CAD build for the part. Positions are in the model's coordinates, mm. A direction names the side the tool comes from. Give positions to 0.01 mm unless a question says otherwise; leave off trailing zeros. Order: outer loops, then holes, each group sorted by start corner. A loop starts at its lowest first (then second) coordinate and runs counter-clockwise, first axis right, second up.
Item 1: Band-saw the part on C-C on z = -0.5. Give the cut face in (x, y).
Item 2: Band-saw the part on D-D on y = 5. Give the cut face in (x, z).
Item 3: Wall check: L1, parallel to Z at x = -1.5, y = -9.5; L2, parallel to Z at x = 4, y = 0.25; L3, parallel to Y at x = -4, z = -4. Give the ranges that are in metal, low to high.
Item 4: Band-saw the part on A-A on y = 0. Give the cut face in (x, z), plus the area to 3 significant figures.
Item 5: Which spindle directions (+Z, -Z, +X, -X, +Y, -Y) get a long thin tool onto all of the face, cutting with end or side? Do faces 1 (the cylindrical face through (1.764, -3.391, 1.377)), 2 (the flat face through (0, 0, -5.588)). Say none if no direction does.
Item 6: Flat gauge pins, fed straight in: P1, Ø2, axis at x = 6.5, z = 0, coming from the +Y side; P2, Ø3, axis at y = -8, z = -2.5, coming from the -X side; P3, Ø1.5, axis at x = -3, z = -4.5, coming from the +Y side; P4, Ø1, axis at y = -6.5, z = 1.5, coming from the -X side. Where does each tip first touch, or does it go through?
```python
from build123d import *

# Parameters (mm, degrees)
F0_R     = 3.8227
F1_DEPTH = 2.794
F0_R_2   = 6.858
F2_DEPTH = 2.794
F3_R     = 11.3665
F3_R_2   = 6.858
F4_DEPTH = 2.794


with BuildPart() as f1:
    # F0 (on Top) → F1 (new body)
    with BuildSketch(Plane.XY):
        Circle(F0_R)
    extrude(amount=F1_DEPTH)

    # F0 (on Top) → F2 (join)
    with BuildSketch(Plane.XY):
        Circle(F0_R_2)
        Circle(F0_R, mode=Mode.SUBTRACT)
        Circle(F0_R)
    extrude(amount=-F2_DEPTH)

    # F3 (on face) → F4 (join)
    with BuildSketch(Plane(origin=(0, 0, -2.794), x_dir=(1, 0, 0), z_dir=(0, 0, -1))):
        Circle(F3_R)
        Circle(F3_R_2, mode=Mode.SUBTRACT)
        Circle(F3_R_2)
    extrude(amount=F4_DEPTH)


solid = f1.part
```
The answers:
1. outline: circle Ø13.72 at (0, 0)
2. outline: (-10.21, -5.59) - (10.21, -5.59) - (10.21, -2.79) - (4.69, -2.79) - (4.69, 0) - (-4.69, 0) - (-4.69, -2.79) - (-10.21, -2.79) - close
3. L1: z = -5.59 to -2.79
3. L2: z = -5.59 to 0
3. L3: y = -10.64 to 10.64
4. outline: (-11.37, -5.59) - (11.37, -5.59) - (11.37, -2.79) - (6.86, -2.79) - (6.86, 0) - (3.82, 0) - (3.82, 2.79) - (-3.82, 2.79) - (-3.82, 0) - (-6.86, 0) - (-6.86, -2.79) - (-11.37, -2.79) - close
4. area: 123 mm2
5. face 1: +Z
5. face 2: -Z, +X, -X, +Y, -Y
6. P1: stops at y = 4.1
6. P2: stops at x = -9.3
6. P3: stops at y = 11.14
6. P4: passes through
